The model under review builds one solid part; all positions refer to its coordinate system, in mm. A direction names the side the tool comes from. Round coordinates to 2 decimals unless told otherwise and drop trailing zeros. Order: outer loops, then holes, each group sorted by start corner. A loop starts at its lowest first (then second) coordinate and runs counter-clockwise, first axis right, second up. Notation, with made-up numbers: M 46,-6 L 99,-6 A24 ccw 99,20 Z; hole C 72.25,-40 d10. An arc over 180 degrees is marked long. Answer as a JSON object with one key per item and string values. Group by question number.
1) Consider section A-A, the plane y = -0.5. Write out the cut boundary in (x, z).
2) The part is to be moulded in two halves that separate along X. For faces 1 (the cylindrical face through (-62.902, -18.266, 0.493)), 2 (the flat face through (-21.091, -14.316, 0.493)), 3 (the flat face through (-41, 27, 0)), say which applies: +X half, -X half, draft (parallel to the pull), parting line (faces both ways), or undercut.
3) Consider section B-B, the plane x = -47. Write out the cut boundary in (y, z), then the cut area to 3 significant figures.
4) Consider section C-C, the plane z = 0.4. Write out the cut boundary in (x, y), then the cut area to 3 significant figures.
5) Insertion check: pin 1 Ø3.5 at (x, y) = (-62.58, -16.8) entering from +Z. The pin has a flat end and moves straight along its axis. Give the tip position at first contact, or say it passes through.
6) To check wall thickness, follow line 1 (Y direction, x = -45, z = 0.25); line 2 (X direction, y = 12.5, z = 0.3); line 3 (Y direction, x = -19, z = 0.8). State the ranges of each line that lie inside material, in increasing order.
7) For faces 4 (the flat face through (-41, 27, 1)), 5 (the flat face through (-60.09, -14.29, 0.49)), list the 3-axis set-ups (+Z, -Z, +X, -X, +Y, -Y) from which the entire face can be reached by the end or side of a thin tool; tool diameter is ignored.
```python
from build123d import *

# Parameters (mm, degrees)
CROQUIS1_W              = 49
CROQUIS1_H              = 49
CROQUIS1_R              = 1.5
SALIENTE_EXTRUIR1_DEPTH = 1


with BuildPart() as part:
    # Croquis1 → Saliente-Extruir1 (new body)
    with BuildSketch(Plane.XY):
        with Locations((-40.576557533, 5.197871677)):
            Rectangle(CROQUIS1_W, CROQUIS1_H)
        with Locations((-62.576557533, 27.197871677)):
            Circle(CROQUIS1_R, mode=Mode.SUBTRACT)
        with Locations((-18.576557533, 27.197871677)):
            Circle(CROQUIS1_R, mode=Mode.SUBTRACT)
        with Locations((-18.576557533, -16.802128323)):
            Circle(CROQUIS1_R, mode=Mode.SUBTRACT)
        with Locations((-62.576557533, -16.802128323)):
            Circle(CROQUIS1_R, mode=Mode.SUBTRACT)
        Polygon((-61.076557533, 23.697871677), (-61.076557533, -13.302128323), (-59.076557533, -15.302128323), (-22.076557533, -15.302128323), (-20.076557533, -13.302128323), (-20.076557533, 23.697871677), (-22.076557533, 25.697871677), (-59.076557533, 25.697871677), align=None, mode=Mode.SUBTRACT)
    extrude(amount=SALIENTE_EXTRUIR1_DEPTH)


solid = part.part
```
Results list:
{
 "1": {"outline": "M -65.08,0 L -61.08,0 L -61.08,1 L -65.08,1 Z; M -20.08,0 L -16.08,0 L -16.08,1 L -20.08,1 Z"},
 "2": {"face 1": "undercut", "face 2": "undercut", "face 3": "draft"},
 "3": {"outline": "M -19.3,0 L -15.3,0 L -15.3,1 L -19.3,1 Z; M 25.7,0 L 29.7,0 L 29.7,1 L 25.7,1 Z", "area": "8.00 mm^2"},
 "4": {"outline": "M -65.08,-19.3 L -16.08,-19.3 L -16.08,29.7 L -65.08,29.7 Z; hole C -62.58,-16.8 d3; hole C -62.58,27.2 d3; hole M -61.08,-13.3 L -59.08,-15.3 L -22.08,-15.3 L -20.08,-13.3 L -20.08,23.7 L -22.08,25.7 L -59.08,25.7 L -61.08,23.7 Z; hole C -18.58,-16.8 d3; hole C -18.58,27.2 d3", "area": "700 mm^2"},
 "5": {"pin 1": "z = 1"},
 "6": {"line 1": "-19.3 to -15.3, 25.7 to 29.7", "line 2": "-65.08 to -61.08, -20.08 to -16.08", "line 3": "-19.3 to -18.24, -15.36 to 25.76, 28.64 to 29.7"},
 "7": {"face 4": "+Z, +X, -X, +Y, -Y", "face 5": "+Z, -Z"}
}
